Here's how the part is built. I have some questions about the finished solid (model axes, mm). A direction names the side the tool comes from. Coordinates: 2 decimals unless noted, no trailing zeros. Write each loop counter-clockwise with the first axis right and the second up, starting at its lowest first coordinate (ties: lowest second). Pieces come first, ordered by that corner, then holes.
Item 1: I want a section at B-B (y = -115.5). Please give me the cut outline in (x, z).
Item 2: I want a section at C-C (x = 1). Please give me the cut outline in (y, z), and give its area (3 significant figures).
Item 3: For faces 1 (the face through (9.86, -123.75, -24.65)), 2 (the face through (10, -133, -36.5)), 3 (the face through (6, -115, -6.5)), which set-ups out of +Z, -Z, +X, -X, +Y, -Y let a thin tool reach every point of the face, with its end or its side?
Item 4: Please list where these lines run through material, in increasing order: line 1 (Z direction, x = 2.35, y = -115.5); line 2 (Z direction, x = 10, y = -134.5); line 3 (X direction, y = -132.5, z = -38.5).
Item 5: I want a section at A-A (x = 10.25). Please give me the cut outline in (y, z).
Item 6: If we mould it in two halves opening along Z, with no side actions, what happens to faces 4 (the face through (2.24, -135.1, -24.65)), 5 (the face through (5.573, -136.366, -10.766))? For each: pulls with the +Z half, pulls with the -Z half, needs draft (parallel to the pull), parting line crosses it, or undercut.
Item 7: I'm going to push flat-ended pins straight in: P1, Ø3, axis at x = 6.5, y = -115, coming from the +Z side; P2, Ø4, axis at x = 11.5, z = -38.5, coming from the -Y side; P3, Ø2, axis at y = -121.5, z = -18, coming from the +X side; P4, Ø1.5, axis at y = -133, z = -43, coming from the +X side. Where does each tip first touch, or does it pass through?
Item 8: I want a section at D-D (y = -122.5). Please give me the cut outline in (x, z), and give its area (3 significant figures).
from build123d import *

# Parameters (mm, degrees)
BOSS_EXTRUDE1_DEPTH = 50
SKETCH2_R           = 2
CUT_EXTRUDE1_DEPTH  = 50
CUT_EXTRUDE2_REACH  = 160.02
SKETCH2_3_R         = 2
SKETCH3_R           = 2
CUT_EXTRUDE3_DEPTH  = 154.134111759
CUT_EXTRUDE4_START  = -6
SKETCH3_3_R         = 2
CUT_EXTRUDE4_DEPTH  = 4


with BuildPart() as part:
    # Sketch1 → Boss-Extrude1 (new body)
    with BuildSketch(Plane.XY):
        Polygon((0, -105.5), (0, -125.5), (4.544210652, -144.976913245), (14.282667274, -142.704807919), (5.313096791, -104.260387197), align=None)
    extrude(amount=-BOSS_EXTRUDE1_DEPTH)

    # Sketch2 → Cut-Extrude1 (cut)
    with BuildSketch(Plane.ZY):
        with Locations((-40, -115.5)):
            Circle(SKETCH2_R)
        with Locations((-10, -115.5)):
            Circle(SKETCH2_R)
    extrude(amount=-CUT_EXTRUDE1_DEPTH, mode=Mode.SUBTRACT)

    # Cut-Extrude2: from a plane face, 160.02 long prism both ways, kept between that surface and its translate by the depth
    cut_extrude2_start = Plane(origin=(14.282667274, -142.704807919, -50), z_dir=(0.9738456622517382, 0.227210532576009, 0)) * Box(642.08, 642.08, 321.04, align=(Align.CENTER, Align.CENTER, Align.MIN), mode=Mode.PRIVATE)
    cut_extrude2_end = Plane(origin=(10.282667274, -142.704807919, -50), z_dir=(0.9738456622517382, 0.227210532576009, 0)) * Box(642.08, 642.08, 321.04, align=(Align.CENTER, Align.CENTER, Align.MIN), mode=Mode.PRIVATE)
    # Sketch2<3> → Cut-Extrude2 (cut, from a surface)
    with BuildSketch(Plane.ZY, mode=Mode.PRIVATE) as cut_extrude2_sk1:
        Polygon((-36.5, -117.520725942), (-36.5, -113.479274058), (-40, -111.458548116), (-43.5, -113.479274058), (-43.5, -117.520725942), (-40, -119.541451884), align=None)
        with Locations((-40, -115.5)):
            Circle(SKETCH2_3_R, mode=Mode.SUBTRACT)
    cut_extrude2_tool1 = extrude(cut_extrude2_sk1.sketch, amount=CUT_EXTRUDE2_REACH, both=True, mode=Mode.PRIVATE)
    add(((cut_extrude2_tool1 - cut_extrude2_start) & cut_extrude2_end).solids().sort_by_distance((5.935441, -115.5, -36.606927))[0], mode=Mode.SUBTRACT)
    # Sketch2<3> → Cut-Extrude2 (cut, from a surface)
    with BuildSketch(Plane.ZY, mode=Mode.PRIVATE) as cut_extrude2_sk2:
        Polygon((-10, -111.458548116), (-6.5, -113.479274058), (-6.5, -117.520725942), (-10, -119.541451884), (-13.5, -117.520725942), (-13.5, -113.479274058), align=None)
        with Locations((-10, -115.5)):
            Circle(SKETCH2_3_R, mode=Mode.SUBTRACT)
    cut_extrude2_tool2 = extrude(cut_extrude2_sk2.sketch, amount=CUT_EXTRUDE2_REACH, both=True, mode=Mode.PRIVATE)
    add(((cut_extrude2_tool2 - cut_extrude2_start) & cut_extrude2_end).solids().sort_by_distance((5.935441, -115.5, -36.606927))[0], mode=Mode.SUBTRACT)

    # Sketch3 → Cut-Extrude3 (cut, through all)
    with BuildSketch(Plane(origin=(-27.769132942, -6.478890577, 0), x_dir=(0, 0, 1), z_dir=(-0.973845662251742, -0.22721053257599275, 0))):
        with Locations(Location((-40, -132.217630613, 0), (0, 0, 270))):
            Circle(SKETCH3_R)
        with Locations(Location((-10, -132.217630613, 0), (0, 0, 270))):
            Circle(SKETCH3_R)
    extrude(amount=-CUT_EXTRUDE3_DEPTH, mode=Mode.SUBTRACT)

    # Sketch3<3> → Cut-Extrude4 (cut)
    # profile 1 of 2: a face of its own
    with BuildSketch(Plane(origin=(-27.769132942, -6.478890577, 0), x_dir=(0, 0, 1), z_dir=(-0.973845662251742, -0.22721053257599275, 0)).offset(CUT_EXTRUDE4_START)):
        Polygon((-36.5, -134.238356555), (-36.5, -130.19690467), (-40, -128.176178728), (-43.5, -130.19690467), (-43.5, -134.238356555), (-40, -136.259082497), align=None)
        with Locations(Location((-40, -132.217630613, 0), (0, 0, 270))):
            Circle(SKETCH3_3_R, mode=Mode.SUBTRACT)
    # profile 2 of 2: a face of its own
    with BuildSketch(Plane(origin=(-27.769132942, -6.478890577, 0), x_dir=(0, 0, 1), z_dir=(-0.973845662251742, -0.22721053257599275, 0)).offset(CUT_EXTRUDE4_START)):
        Polygon((-10, -128.176178728), (-6.5, -130.19690467), (-6.5, -134.238356555), (-10, -136.259082497), (-13.5, -134.238356555), (-13.5, -130.19690467), align=None)
        with Locations(Location((-10, -132.217630613, 0), (0, 0, 270))):
            Circle(SKETCH3_3_R, mode=Mode.SUBTRACT)
    extrude(amount=-CUT_EXTRUDE4_DEPTH, mode=Mode.SUBTRACT)


solid = part.part
Answer:
1. outline: (0, -50) - (7.94, -50) - (7.94, -43.5) - (3.94, -43.5) - (3.94, -42) - (0, -42) - close; (0, -38) - (3.94, -38) - (3.94, -36.5) - (7.94, -36.5) - (7.94, -13.5) - (3.94, -13.5) - (3.94, -12) - (0, -12) - close; (0, -8) - (3.94, -8) - (3.94, -6.5) - (7.94, -6.5) - (7.94, 0) - (0, 0) - close
2. outline: (-129.79, -50) - (-105.27, -50) - (-105.27, 0) - (-129.79, 0) - close; hole circle Ø4 at (-115.5, -40); hole circle Ø4 at (-115.5, -10)
2. area: 1,200 mm2
3. face 1: +Z, -Z, +X, +Y
3. face 2: none
3. face 3: +X
4. line 1: z = -50 to -42, -38 to -12, -8 to 0
4. line 2: z = -50 to -43.5, -36.5 to -13.5, -6.5 to 0
4. line 3: x = 1.63 to 7.79
5. outline: (-143.65, -50) - (-125.42, -50) - (-125.42, 0) - (-143.65, 0) - close; hole (-137.53, -40) - (-135.45, -43.5) - (-131.3, -43.5) - (-129.23, -40) - (-131.3, -36.5) - (-135.45, -36.5) - close; hole (-137.53, -10) - (-135.45, -13.5) - (-131.3, -13.5) - (-129.23, -10) - (-131.3, -6.5) - (-135.45, -6.5) - close
6. face 4: needs draft
6. face 5: undercut
7. P1: stops at z = 0
7. P2: stops at y = -143.82
7. P3: stops at x = 9.57
7. P4: stops at x = 12.15
8. outline: (0, -50) - (9.57, -50) - (9.57, 0) - (0, 0) - close
8. area: 478 mm2
